Input: part model. Units: mm. Frame: model coordinates. A direction names the side the tool comes from. Round coordinates to 2 decimals unless told otherwise and drop trailing zeros. Loops run counter-clockwise (first coordinate to the right, second up) from the corner with the lowest first, then second, coordinate; pieces in that order, holes last. Notation, with made-up numbers: (-22, 88.25) -> (11, 88.25) arc R7 ccw to (11, 99.25) -> close; hole circle Ø10 at (25.25, 59.25). An arc over 180 degrees is marked (long way). One line per question, with ' | ' between items. Start each with the question number.
Q1. Contact query for a flat-ended pin moving along its axis: P1, Ø2.5, axis at x = 161, z = 7, coming from the -Y side. Output: stop coordinate, or through.
Q2. Cut plane A-A on x = 74. Return loops of the section in (y, z), and give its area (3 significant figures).
Q3. Access query for faces 4 (the face through (164.2, 68.6, 9)), 5 (the face through (99, 100, 7)), 6 (the face through (42.31, 12.32, 6.54)). Directions: +Z, -Z, +X, -X, +Y, -Y. A direction counts if a zero-diameter tool reaches every point of the face in a straight line with its end or side. Return the directions, or none.
Q4. Mould query, pull axis Y, two halves, no side actions, for faces 1 (the face through (40, 25, 8)), 2 (the face through (78, 12, 6)), 3 (the face through (120.805, 39.029, 12.042)). Classes: pulls with the +Y half, pulls with the -Y half, needs draft (parallel to the pull), parting line crosses it, or undercut.
Q5. Cut plane B-B on y = 70.8. State how many separate pieces and enclosed holes the cut face has, and give its area (3 significant figures).
Q6. Material intervals for L1, parallel to Y at x = 162, z = 2.5; L2, parallel to Y at x = 38, z = 11.45; L3, parallel to X at y = 11, z = 8.5, sorted ascending.
from build123d import *

# Parameters (mm, degrees)
SKETCH_W        = 200
SKETCH_H        = 100
PAD_DEPTH       = 15
SKETCH001_R     = 2.75
POCKET_DEPTH    = 15
SKETCH002_R     = 5.2
POCKET001_DEPTH = 6
SKETCH003_R     = 2.5
POCKET002_DEPTH = 25


with BuildPart() as part:
    # Sketch → Pad (new body)
    with BuildSketch(Plane.XY):
        with Locations((100, 50)):
            Rectangle(SKETCH_W, SKETCH_H)
    extrude(amount=PAD_DEPTH)

    # Sketch001 (on Face6 of Pad) → Pocket (cut)
    with BuildSketch(Plane.XY.offset(15)):
        with Locations((162, 70.8)):
            Circle(SKETCH001_R)
        with Locations((162, 38.8)):
            Circle(SKETCH001_R)
        with Locations((126, 70.8)):
            Circle(SKETCH001_R)
        with Locations((126, 38.8)):
            Circle(SKETCH001_R)
        with Locations((74, 70.8)):
            Circle(SKETCH001_R)
        with Locations((74, 38.8)):
            Circle(SKETCH001_R)
        with Locations((38, 70.8)):
            Circle(SKETCH001_R)
        with Locations((38, 38.8)):
            Circle(SKETCH001_R)
    extrude(amount=-POCKET_DEPTH, mode=Mode.SUBTRACT)

    # Sketch002 (on Face5 of Pocket) → Pocket001 (cut)
    with BuildSketch(Plane.XY.offset(15)):
        with Locations((38, 70.8)):
            Circle(SKETCH002_R)
        with Locations((38, 38.8)):
            Circle(SKETCH002_R)
        with Locations((74, 70.8)):
            Circle(SKETCH002_R)
        with Locations((74, 38.8)):
            Circle(SKETCH002_R)
        with Locations((126, 70.8)):
            Circle(SKETCH002_R)
        with Locations((126, 38.8)):
            Circle(SKETCH002_R)
        with Locations((162, 70.8)):
            Circle(SKETCH002_R)
        with Locations((162, 38.8)):
            Circle(SKETCH002_R)
    extrude(amount=-POCKET001_DEPTH, mode=Mode.SUBTRACT)

    # Sketch003 (on Face6 of Pocket001) → Pocket002 (cut)
    with BuildSketch(Plane.XZ):
        with Locations((40, 7.5)):
            Circle(SKETCH003_R)
        with Locations((80, 7.5)):
            Circle(SKETCH003_R)
        with Locations((120, 7.5)):
            Circle(SKETCH003_R)
        with Locations((160, 7.5)):
            Circle(SKETCH003_R)
    extrude(amount=-POCKET002_DEPTH, mode=Mode.SUBTRACT)


solid = part.part
Results:
1) P1: y = 25
2) outline: (0, 0) -> (36.05, 0) -> (36.05, 9) -> (33.6, 9) -> (33.6, 15) -> (0, 15) -> close; (41.55, 0) -> (68.05, 0) -> (68.05, 9) -> (65.6, 9) -> (65.6, 15) -> (44, 15) -> (44, 9) -> (41.55, 9) -> close; (73.55, 0) -> (100, 0) -> (100, 15) -> (76, 15) -> (76, 9) -> (73.55, 9) -> close | area: 1,280 mm^2
3) face 4: +Z | face 5: +Z, -Z, +X, -X, +Y | face 6: -Y
4) face 1: pulls with the -Y half | face 2: needs draft | face 3: undercut
5) separate pieces: 5 | enclosed holes: 0 | area: 2,550 mm^2
6) L1: 0 to 36.05, 41.55 to 68.05, 73.55 to 100 | L2: 0 to 33.6, 44 to 65.6, 76 to 100 | L3: 0 to 37.71, 42.29 to 77.71, 82.29 to 117.71, 122.29 to 157.71, 162.29 to 200
